Design review of the part shown in the three views and the two pictorial views. Dimensions are in mm from the part's minimum x, y and z. Round coordinates to 2 decimals unless told otherwise and drop trailing zeros. Write each loop counter-clockwise with the first axis right and the second up, starting at its lowest first coordinate (ties: lowest second). Pieces come first, ordered by that corner, then holes. Notation, with made-up numbers: (52, 52.5) -> (100, 52.5) arc R27 cw to (100, 76.5) -> close; hole circle Ø4 at (85, -21). An arc over 180 degrees is marked (long way). Return JSON: item names as keys, results as strings. Group by question number.
1. Clearance check with a flat-ended pin moving along its axis: P1, Ø0.8, axis at y = 0.5, z = 1, coming from the -X side. State where the tip first meets the part, or that it passes through.
2. For line 1 along Z through (x, y) = (13, 0.9); line 2 along X through (y, z) = (0.5, 1.25), list the stretches that pass through material, from the lowest coordinate up. Write a range as from..to.
3. Take a section at B-B, the plane x = 33. Write out the cut boundary in (y, z), then the cut area to 3 significant figures.
4. Take a section at C-C, the plane z = 15.5. Write out the cut boundary in (x, y), then the cut area to 3 significant figures.
5. Take a section at A-A, the plane y = 0.3. Write out the cut boundary in (x, z).
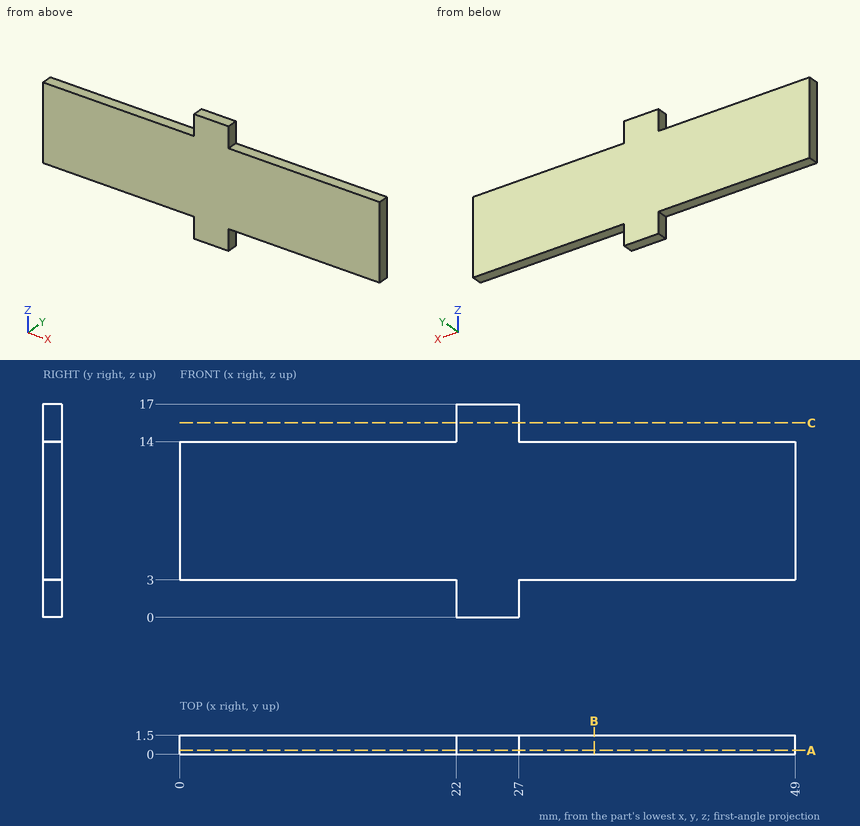
Output:
{
 "1": {"P1": "stops at x = 22"},
 "2": {"line 1": "z = 3..14", "line 2": "x = 22..27"},
 "3": {"outline": "(0, 3) -> (1.5, 3) -> (1.5, 14) -> (0, 14) -> close", "area": "16.5 mm^2"},
 "4": {"outline": "(22, 0) -> (27, 0) -> (27, 1.5) -> (22, 1.5) -> close", "area": "7.50 mm^2"},
 "5": {"outline": "(0, 3) -> (22, 3) -> (22, 0) -> (27, 0) -> (27, 3) -> (49, 3) -> (49, 14) -> (27, 14) -> (27, 17) -> (22, 17) -> (22, 14) -> (0, 14) -> close"}
}
